Autodesk Inventor part; units mm, degrees
ref_plane "Plano de trabalho1" through (0, 0, -6) normal (0, 0, 1) x (1, 0, 0)
ref_plane "Plano de trabalho2" through (0, 0, -6) normal (0, 0, 1) x (1, 0, 0)
ref_plane "Plano de trabalho3" through (0, 0, 6) normal (0, 0, 1) x (1, 0, 0)
sketch "Esboço1" plane through (0, 0, 0) normal (0, 1, 0) x (-1, 0, 0)
  circle A0 centre (0, 0) radius 6
  dimension "d0" = 12
extrude "Extrusão1" add sketch "Esboço1" along normal blind 88
ref_plane "Plano de trabalho1" through (0, 0, -6) normal (0, 0, 1) x (1, 0, 0)
ref_plane "Plano de trabalho2" through (0, 0, -6) normal (0, 0, 1) x (1, 0, 0)
ref_plane "Plano de trabalho3" through (0, 0, 6) normal (0, 0, 1) x (1, 0, 0)
sketch "Esboço2" plane through (0, 0, -6) normal (0, 0, 1) x (1, 0, 0)
  line L0 (0, 92.3715) -> (0, -4.0857) construction
  line L1 (-6, 0) -> (-6, 88) construction
  line L2 (-6, 88) -> (-6, 58) construction
  line L3 (-6, 58) -> (-6, 48) construction
  line L4 (0, 58) -> (0, 48) construction
  line L5 (-1.25, 58) -> (-1.25, 48)
  line L6 (1.25, 48) -> (1.25, 58)
  arc A0 (1.25, 58) -> (-1.25, 58) centre (0, 58) ccw
  arc A1 (-1.25, 48) -> (1.25, 48) centre (0, 48) ccw
  line L7 (-6, 0) -> (-6, 10) construction
  line L8 (0, 10) -> (0, 0) construction
  line L9 (-1.25, 10) -> (-1.25, 0)
  line L10 (1.25, 0) -> (1.25, 10)
  arc A2 (1.25, 10) -> (-1.25, 10) centre (0, 10) ccw
  arc A3 (-1.25, 0) -> (1.25, 0) centre (0, 0) ccw
  point P0 (0, 53)
  point P1 (0, 5)
  dimension "d4" = 30
  dimension "d5" = 10
  dimension "d6" = 2.5
  dimension "d7" = 10
  dimension "d8" = 2.5
extrude "Extrusão2" cut sketch "Esboço2" along normal blind 2.5
properties part number "eixo 4"
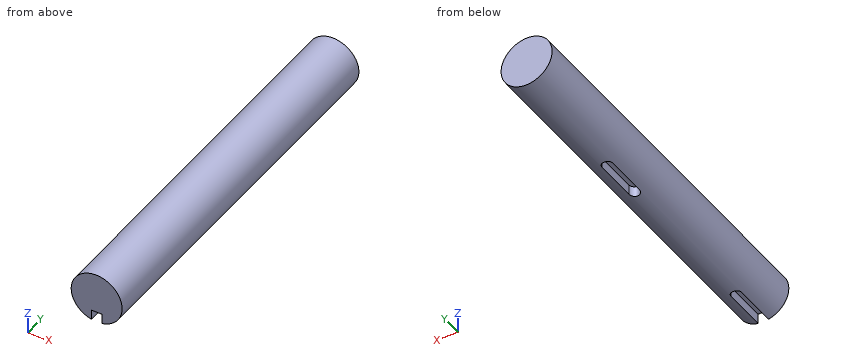
The model under review builds one solid part; all positions refer to its coordinate system, in mm. Give positions to 0.01 mm unless a question says otherwise; leave off trailing zeros. Loops run counter-clockwise (first coordinate to the right, second up) from the corner with the lowest first, then second, coordinate; pieces in that order, holes last. Notation, with made-up numbers: (-12.5, 65) -> (28.5, 65) arc R16 cw to (28.5, 81) -> close; hole circle Ø10 at (83.5, -4.5). An arc over 180 degrees is marked (long way). Answer as a JSON object with one key per item and string values. Group by question number.
Q1. Wall thickness on line 1 along Z through (x, y) = (-0.25, 33.5); line 2 along Y through (x, z) = (0.25, -5.25): over which ranges is each line inside the solid? List them lowest first.
Q2. Take a section at A-A (x = 0). Write out the cut boundary in (y, z), plus the area to 3 significant figures.
Q3. Take a section at D-D (z = 3.5). Write out the cut boundary in (x, y).
Q4. Insertion check: pin 1 (0.7 mm diameter, centred on y = 5.5, z = -4.5, fed in from +X); pin 2 (0.7 mm diameter, centred on y = 54.5, z = -5, fed in from -X); pin 3 (2.5 mm diameter, centred on y = 52, z = -5, fed in from +X). Each pin has a flat end and moves straight along its axis. Give the tip position at first contact, or say it passes through.
Q5. Take a section at B-B (y = 40.5). Write out the cut boundary in (x, z).
Q6. Take a section at C-C (z = -4.25). Write out the cut boundary in (x, y).
Answer below:
{
 "1": {"line 1": "z = -5.99 to 5.99", "line 2": "y = 11.22 to 46.78, 59.22 to 88"},
 "2": {"outline": "(0, -3.5) -> (11.25, -3.5) -> (11.25, -6) -> (46.75, -6) -> (46.75, -3.5) -> (59.25, -3.5) -> (59.25, -6) -> (88, -6) -> (88, 6) -> (0, 6) -> close", "area": "997 mm2"},
 "3": {"outline": "(-4.87, 0) -> (4.87, 0) -> (4.87, 88) -> (-4.87, 88) -> close"},
 "4": {"pin 1": "stops at x = 4.33", "pin 2": "stops at x = -3.79", "pin 3": "stops at x = 4.68"},
 "5": {"outline": "circle Ø12 at (0, 0)"},
 "6": {"outline": "(-4.24, 0) -> (-1.25, 0) -> (-1.25, 10) arc R1.25 cw to (1.25, 10) -> (1.25, 0) -> (4.24, 0) -> (4.24, 88) -> (-4.24, 88) -> close; hole (-1.25, 48) arc R1.25 ccw to (1.25, 48) -> (1.25, 58) arc R1.25 ccw to (-1.25, 58) -> close"}
}
